Input: part model. Units: mm. Frame: model coordinates. Face numbers are marked on the shaded views. Coordinates: 2 decimals unless noted, no trailing zeros. Write each loop counter-clockwise with the first axis right and the second up, starting at its lowest first coordinate (ties: lowest second). Pieces come first, ordered by that corner, then holes. Notation, with made-up numbers: M -15,59.5 L 31,59.5 A23 cw 31,90.5 Z; hole C 46,87 d9. An arc over 180 degrees is marked long. Use CSV: the item, a comma, the result in double quotes.
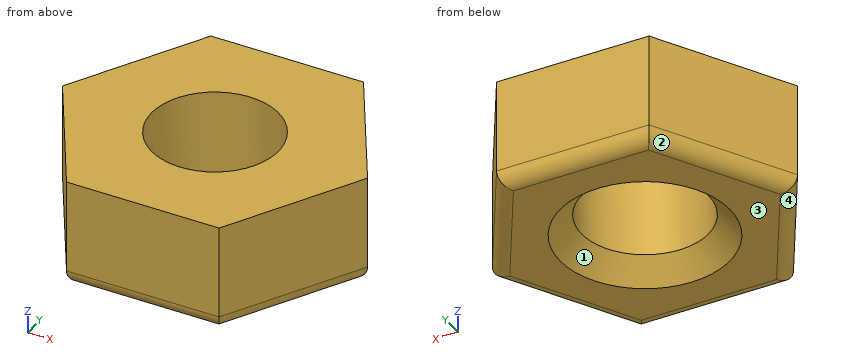
```python
from build123d import *

# Parameters (mm, degrees)
F1_DEPTH       = 1.085
F3_D           = 2.54
F3_CSINK_D     = 3.4
F3_CSINK_ANGLE = 90
F4_R           = 0.3


with BuildPart() as f1:
    # F0 (on Top) → F1 (new body, symmetric)
    with BuildSketch(Plane.XY):
        Polygon((1.524205, -2.64), (3.048409, 0), (1.524205, 2.64), (-1.524205, 2.64), (-3.048409, 0), (-1.524205, -2.64), align=None)
    extrude(amount=F1_DEPTH, both=True)

    # F3 (through all)
    with Locations(Plane(origin=(0, 0, -1.085), x_dir=(1, 0, 0), z_dir=(0, 0, -1))):
        with Locations((0, 0)):
            CounterSinkHole(F3_D / 2, F3_CSINK_D / 2, counter_sink_angle=F3_CSINK_ANGLE)

    # F4
    f4_edges = [f1.edges().sort_by_distance(p)[0] for p in [
        (2.286307, 1.32, -1.085),
        (2.286307, -1.32, -1.085),
        (0, -2.64, -1.085),
        (-2.286307, -1.32, -1.085),
        (-2.286307, 1.32, -1.085),
        (0, 2.64, -1.085),
    ]]
    fillet(f4_edges, radius=F4_R)


solid = f1.part
```
1. Mould query, pull axis Y, two halves, no side actions, for the marked faces 1, 2, 3 and 4. Classes: pulls with the +Y half, pulls with the -Y half, needs draft (parallel to the pull), parting line crosses it, or undercut.
Resolved:
face 1,"undercut"
face 2,"pulls with the +Y half"
face 3,"needs draft"
face 4,"pulls with the -Y half"
2. Section A-A (x = 0). Return loops of the section in (y, z) (3 decimals).
Resolved:
outline,"M -2.64,-0.785 A0.3 ccw -2.34,-1.085 L -1.7,-1.085 L -1.27,-0.655 L -1.27,1.085 L -2.64,1.085 Z; M 1.27,-0.655 L 1.7,-1.085 L 2.34,-1.085 A0.3 ccw 2.64,-0.785 L 2.64,1.085 L 1.27,1.085 Z"
3. Section B-B (z = 0.15). Return loops of the section in (x, y).
Resolved:
outline,"M -3.05,0 L -1.52,-2.64 L 1.52,-2.64 L 3.05,0 L 1.52,2.64 L -1.52,2.64 Z; hole C 0,0 d2.54"
4. Material intervals for line 1 (Y direction, x = 0, z = -0.25); line 2 (X direction, y = -0.2, z = -0.1); line 3 (X direction, y = 0.95, z = 0.6), sorted ascending. Write a range as [from, to].
Resolved:
line 1,"y = [-2.64, -1.27], [1.27, 2.64]"
line 2,"x = [-2.93, -1.25], [1.25, 2.93]"
line 3,"x = [-2.5, -0.84], [0.84, 2.5]"
